Read the model definition and answer for the solid it produces. Units are mm, in the model's axes. Face numbers are marked on the shaded views. A direction names the side the tool comes from. Coordinates: 2 decimals unless noted, no trailing zeros. Order: outer loops, then holes, each group sorted by start corner. A loop starts at its lowest first (then second) coordinate and runs counter-clockwise, first axis right, second up. Notation, with made-up numbers: (10.5, -18.5) - (49.5, -18.5) arc R37 cw to (49.5, 19.5) - close; hole circle Ø5 at (14.5, 81). An arc over 180 degrees is marked (long way). Use one line per item in the form item = value.
```python
from build123d import *

# Parameters (mm, degrees)
Y_KSEKLIK_EKSTR_ZYON1_DEPTH = 50
Y_KSEKLIK_EKSTR_ZYON2_DEPTH = 7.5


with BuildPart() as part:
    # Çizim1 → Yükseklik-Ekstrüzyon1 (new body)
    with BuildSketch(Plane.XY):
        with BuildLine():
            Line((-7.5, 12.5), (7.5, 12.5))
            ThreePointArc((7.5, 12.5), (11.035533906, 11.035533906), (12.5, 7.5))
            Line((12.5, 7.5), (12.5, -7.5))
            ThreePointArc((12.5, -7.5), (11.035533906, -11.035533906), (7.5, -12.5))
            Line((7.5, -12.5), (-7.5, -12.5))
            ThreePointArc((-7.5, -12.5), (-11.035533906, -11.035533906), (-12.5, -7.5))
            Line((-12.5, -7.5), (-12.5, 7.5))
            ThreePointArc((-12.5, 7.5), (-11.035533906, 11.035533906), (-7.5, 12.5))
        make_face()
    extrude(amount=Y_KSEKLIK_EKSTR_ZYON1_DEPTH)

    # Çizim2 → Yükseklik-Ekstrüzyon2 (add)
    with BuildSketch(Plane.XY):
        with BuildLine():
            Line((1.75, 3.75), (-1.75, 3.75))
            ThreePointArc((-1.75, 3.75), (-3.164213562, 3.164213562), (-3.75, 1.75))
            Line((-3.75, 1.75), (-3.75, -1.75))
            ThreePointArc((-3.75, -1.75), (-3.164213562, -3.164213562), (-1.75, -3.75))
            Line((-1.75, -3.75), (1.75, -3.75))
            ThreePointArc((1.75, -3.75), (3.164213562, -3.164213562), (3.75, -1.75))
            Line((3.75, -1.75), (3.75, 1.75))
            ThreePointArc((3.75, 1.75), (3.164213562, 3.164213562), (1.75, 3.75))
        make_face()
    extrude(amount=-Y_KSEKLIK_EKSTR_ZYON2_DEPTH)


solid = part.part
```
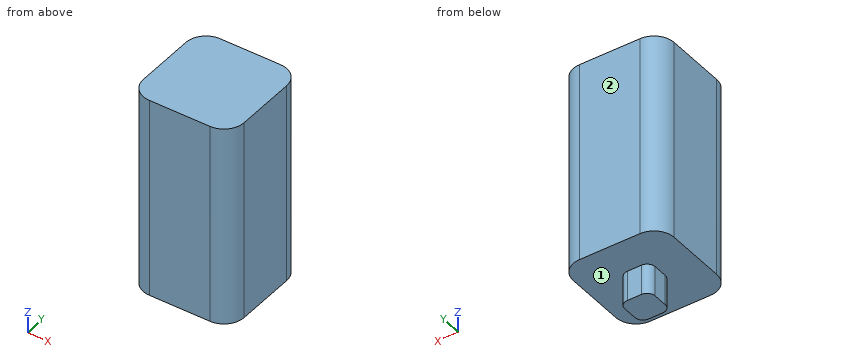
(1) Section D-D, the plane y = -6 is taken. Write down the section's boundary in (x, z).
Answer list:
outline = (-12.5, 0) - (12.5, 0) - (12.5, 50) - (-12.5, 50) - close
(2) Section C-C, the plane x = 8.5 is taken. Write down the section's boundary in (y, z), then the cut area to 3 significant figures.
Answer list:
outline = (-12.4, 0) - (12.4, 0) - (12.4, 50) - (-12.4, 50) - close
area = 1,240 mm2
(3) Which of the six approach directions +Z, -Z, +X, -X, +Y, -Y give full straight-line access (tool end or side, diameter ignored) to the marked faces 1 and 2?
Answer list:
face_1 = -Z
face_2 = +Z, -Z, +X, -X, +Y
(4) Given pin 1 Ø10 at (x, y) = (-8, -9) entering from -Z; pin 2 Ø3 at (x, z) = (0.5, -3) entering from -Y; pin 3 Ø1.8 at (y, z) = (1, -3) entering from -X, each flat-ended and moving along its own axis, determine where each tip first touches the part or whether it passes through.
Answer list:
pin_1 = 0
pin_2 = -3.75
pin_3 = -3.75
(5) Straight lines are drawn through the part: L1, parallel to Z at x = -5.25, y = -5; L2, parallel to Y at x = -1.75, z = -3.5. For each, find the intervals that lie inside material, in ascending order.
Answer list:
L1 = 0 to 50
L2 = -3.75 to 3.75
(6) Section A-A, the plane z = 45.5 is taken. Write down the section's boundary in (x, y).
Answer list:
outline = (-12.5, -7.5) arc R5 ccw to (-7.5, -12.5) - (7.5, -12.5) arc R5 ccw to (12.5, -7.5) - (12.5, 7.5) arc R5 ccw to (7.5, 12.5) - (-7.5, 12.5) arc R5 ccw to (-12.5, 7.5) - close
(7) Section B-B, the plane y = 3 is taken. Write down the section's boundary in (x, z), then the cut area to 3 significant figures.
Answer list:
outline = (-12.5, 0) - (-3.31, 0) - (-3.31, -7.5) - (3.31, -7.5) - (3.31, 0) - (12.5, 0) - (12.5, 50) - (-12.5, 50) - close
area = 1,300 mm2
